```python
from build123d import *

# Parameters (mm, degrees)
SCHIZZO1_W                   = 35
SCHIZZO1_H                   = 45
SCHIZZO1_R                   = 7.6
ESTRUSIONE_ESTRUSIONE1_DEPTH = 35
SCHIZZO3_R                   = 7.6
TAGLIO_ESTRUSIONE1_DEPTH     = 35
RACCORDO1_R                  = 1


with BuildPart() as part:
    # Schizzo1 → Estrusione-Estrusione1 (new body)
    with BuildSketch(Plane.XY):
        with Locations((0.121961372, 0)):
            Rectangle(SCHIZZO1_W, SCHIZZO1_H)
        with Locations((0, -11.15)):
            Circle(SCHIZZO1_R, mode=Mode.SUBTRACT)
    extrude(amount=ESTRUSIONE_ESTRUSIONE1_DEPTH)

    # Schizzo3 → Taglio-Estrusione1 (cut)
    with BuildSketch(Plane(origin=(17.621961372, 0, 0), x_dir=(0, 0, -1), z_dir=(1, 0, 0))):
        with Locations(Location((-17.5, 11.15, 0), (0, 0, 90))):
            Circle(SCHIZZO3_R)
    extrude(amount=-TAGLIO_ESTRUSIONE1_DEPTH, mode=Mode.SUBTRACT)

    # Raccordo1
    raccordo1_edges = [part.edges().sort_by_distance(p)[0] for p in [
        (17.621961372, 0, 35),
        (0.121961372, 22.5, 35),
        (-17.378038628, 0, 35),
        (0.121961372, 22.5, 0),
        (17.621961372, 0, 0),
        (0.121961372, -22.5, 0),
        (-17.378038628, 0, 0),
        (0.121961372, -22.5, 35),
        (-17.378038628, 22.5, 17.5),
        (17.621961372, 22.5, 17.5),
        (17.621961372, -22.5, 17.5),
        (-17.378038628, -22.5, 17.5),
    ]]
    fillet(raccordo1_edges, radius=RACCORDO1_R)


solid = part.part
```
Check sheet for the modelled part. Datum: model origin and axes. Units: mm. Coordinates: 2 decimals unless noted, no trailing zeros. Loops run counter-clockwise (first coordinate to the right, second up) from the corner with the lowest first, then second, coordinate; pieces in that order, holes last.
1) Sectioned sample at C-C (x = 0). Record the boundary of the cut face in (y, z).
2) Gauge pin test, flat ends, axial feed: pin 1 (20 mm diameter, centred on y = 11.15, z = 17.5, fed in from -X); pin 2 (2 mm diameter, centred on x = 3, y = -5.5, fed in from +Z). Record the tip position at first contact, or that the pin passes through.
3) Sectioned sample at A-A (y = 11.15). Record the boundary of the cut face in (x, z).
4) Sectioned sample at D-D (z = 12). Record the boundary of the cut face in (x, y) (3 decimals), and give its area (3 significant figures).
5) Release check for a two-part mould opening along Y. For faces 1 (the face through (0, 0, 35)), 2 (the face through (0, 22.5, 17)), 3 (the face through (0.367, 15.236, 23.908)) record: released by +Y, released by -Y, zero draft, split by the parting line, or undercut.
6) Material ranges on probe 1 along Z at (x, y) = (2, 11.15); probe 2 along Y at (x, z) = (6, 24); probe 3 along X at (y, z) = (-11.5, 7.5), recorded low to high.
7) Sectioned sample at B-B (x = 9). Record the boundary of the cut face in (y, z).
Check sheet entries:
1. outline: (-22.5, 1) arc R1 ccw to (-21.5, 0) - (-18.75, 0) - (-18.75, 35) - (-21.5, 35) arc R1 ccw to (-22.5, 34) - close; (-3.55, 0) - (21.5, 0) arc R1 ccw to (22.5, 1) - (22.5, 34) arc R1 ccw to (21.5, 35) - (-3.55, 35) - close; hole circle Ø15.2 at (11.15, 17.5)
2. pin 1: stops at x = -17.38
2. pin 2: passes through
3. outline: (-17.38, 1) arc R1 ccw to (-16.38, 0) - (16.62, 0) arc R1 ccw to (17.62, 1) - (17.62, 9.9) - (-17.38, 9.9) - close; (-17.38, 25.1) - (17.62, 25.1) - (17.62, 34) arc R1 ccw to (16.62, 35) - (-16.38, 35) arc R1 ccw to (-17.38, 34) - close
4. outline: (-17.378, -21.5) arc R1 ccw to (-16.378, -22.5) - (16.622, -22.5) arc R1 ccw to (17.622, -21.5) - (17.622, 5.905) - (-17.378, 5.905) - close; (-17.378, 16.395) - (17.622, 16.395) - (17.622, 21.5) arc R1 ccw to (16.622, 22.5) - (-16.378, 22.5) arc R1 ccw to (-17.378, 21.5) - close; hole circle Ø15.2 at (0, -11.15)
4. area: 1,030 mm2
5. face 1: zero draft
5. face 2: released by +Y
5. face 3: undercut
6. probe 1: z = 0 to 9.9, 25.1 to 35
6. probe 2: y = -22.5 to -15.81, -6.49 to 7.21, 15.09 to 22.5
6. probe 3: x = -17.38 to -7.59, 7.59 to 17.62
7. outline: (-22.5, 1) arc R1 ccw to (-21.5, 0) - (21.5, 0) arc R1 ccw to (22.5, 1) - (22.5, 34) arc R1 ccw to (21.5, 35) - (-21.5, 35) arc R1 ccw to (-22.5, 34) - close; hole circle Ø15.2 at (11.15, 17.5)
